Verification items for the finished model (mm, model axes). A direction names the side the tool comes from. Coordinates: 2 decimals unless noted, no trailing zeros. Answer as CSV lines item,"result". Start each with the question number.
1. Mould release check, pull along Y, two halves, no side actions. Record for faces 1 (the flat face through (45, -42.679, -10)), 2 (the flat face through (20, -66, -50.8)), 3 (the cylindrical face through (11.75, -57.24, 6.37)): pulls with the +Y half, pulls with the -Y half, needs draft (parallel to the pull), parting line crosses it, or undercut.
2. Set-up check for faces 4 (the cylindrical face through (11.569, -65.792, 6.368)), 5 (the flat face through (16.233, -34, -45)), 6 (the flat face through (3, -61.729, -58)), 7 (the cylindrical face through (19.898, -68.856, 10.196)): record each of +Z, -Z, +X, -X, +Y, -Y from which the full face is reachable in a straight line by a thin tool's end or side.
3. Section check A-A (y = -59.5). Count the separate pieces of the cut face and the enclosed holes in it, and give its area (3 significant figures).
4. Go/stop test with flat-tipped pins: pin 1 (8.5 mm diameter, centred on x = 46, z = -13, fed in from -Y); pin 2 (3.5 mm diameter, centred on x = 28.93, y = -29.98, fed in from -Z); pin 3 (3.5 mm diameter, centred on x = 18.5, y = -66.5, fed in from +Z); pin 4 (6 mm diameter, centred on x = 24.5, z = -47, fed in from -Y). Record where each tip stops, or that it passes through.
5. Material ranges on L1, parallel to Y at x = 25, z = -46.5; L2, parallel to X at y = -54, z = -55; L3, parallel to Z at x = 7.5, y = -51.5, recorded low to high. Write a range as [from, to].
from build123d import *

# Parameters (mm, degrees)
SKETCH1_W            = 50.8
SKETCH1_H            = 76.2
BOSS_EXTRUDE1_DEPTH  = 12.7
SKETCH3_R            = 2.032
CUT_EXTRUDE1_DEPTH   = 12.7
SKETCH17_W           = 7.62
SKETCH17_H           = 76.2
BOSS_EXTRUDE13_DEPTH = 68.58
SKETCH18_W           = 3.81
SKETCH18_H           = 19.05
BOSS_EXTRUDE14_DEPTH = 43.18
SKETCH19_W           = 29.21
SKETCH19_H           = 19.05
BOSS_EXTRUDE15_DEPTH = 43.18
SKETCH4_R            = 4.064
CUT_EXTRUDE5_DEPTH   = 125.729995039
CUT_EXTRUDE6_START   = -5.08
SKETCH21_R           = 11.176
SKETCH21_R_2         = 4.064
CUT_EXTRUDE6_DEPTH   = 5.08
SKETCH22_R           = 11.176
SKETCH22_R_2         = 4.064
CUT_EXTRUDE7_DEPTH   = 5.08
SKETCH23_W           = 19.05
SKETCH23_H           = 38.1
CUT_EXTRUDE8_DEPTH   = 115.424594585
SKETCH26_W           = 17.78
SKETCH26_H           = 46.99
BOSS_EXTRUDE16_DEPTH = 57.15
SKETCH28_W           = 50.8
SKETCH28_H           = 81.28
BOSS_EXTRUDE18_DEPTH = 3.81
SKETCH35_R           = 4.064
CUT_EXTRUDE10_DEPTH  = 125.729995039
SKETCH32_R           = 2.032
CUT_EXTRUDE12_DEPTH  = 9.525
SKETCH41_R           = 2.032
CUT_EXTRUDE14_DEPTH  = 9.525
SKETCH43_R           = 3.96875
CUT_EXTRUDE15_DEPTH  = 4.7625
SKETCH46_R           = 3.937
CUT_EXTRUDE17_DEPTH  = 3.048
SKETCH48_R           = 2.54
CUT_EXTRUDE18_DEPTH  = 25.908
SKETCH49_W           = 50.8
SKETCH49_H           = 4.744734857
CUT_EXTRUDE19_DEPTH  = 92.202
CUT_EXTRUDE20_DEPTH  = 92.202
SKETCH52_W           = 50.8
SKETCH52_H           = 6.844747076
CUT_EXTRUDE21_DEPTH  = 62.484
CUT_EXTRUDE22_DEPTH  = 23.876
FILLET1_R            = 6.35
FILLET2_R            = 6.35
FILLET3_R            = 6.35
FILLET4_R            = 6.35
FILLET5_R            = 6.35
FILLET6_R            = 6.35
FILLET7_R            = 6.35
FILLET8_R            = 6.35


with BuildPart() as part:
    # Sketch1 → Boss-Extrude1 (new body)
    with BuildSketch(Plane.XY):
        with Locations((23.853164533, -42.679075546)):
            Rectangle(SKETCH1_W, SKETCH1_H)
    extrude(amount=BOSS_EXTRUDE1_DEPTH)

    # Sketch3 → Cut-Extrude1 (cut)
    with BuildSketch(Plane.XY.offset(12.7)):
        with Locations((28.933164533, -42.679075546)):
            Circle(SKETCH3_R)
        with Locations((28.933164533, -29.979075546)):
            Circle(SKETCH3_R)
        with Locations((28.933164533, -17.279075546)):
            Circle(SKETCH3_R)
    extrude(amount=-CUT_EXTRUDE1_DEPTH, mode=Mode.SUBTRACT)

    # Sketch17 → Boss-Extrude13 (add)
    with BuildSketch(Plane(origin=(0, 0, 0), x_dir=(-1, 0, 0), z_dir=(0, 0, -1))):
        with Locations((-45.443164533, -42.679075546)):
            Rectangle(SKETCH17_W, SKETCH17_H)
    extrude(amount=BOSS_EXTRUDE13_DEPTH)

    # Sketch18 → Boss-Extrude14 (add)
    with BuildSketch(Plane.ZY.offset(-41.633164533)):
        with Locations((-66.675, -71.254075546)):
            Rectangle(SKETCH18_W, SKETCH18_H)
    extrude(amount=BOSS_EXTRUDE14_DEPTH)

    # Sketch19 → Boss-Extrude15 (add)
    with BuildSketch(Plane.ZY.offset(-41.633164533)):
        with Locations((-36.195, -71.254075546)):
            Rectangle(SKETCH19_W, SKETCH19_H)
    extrude(amount=BOSS_EXTRUDE15_DEPTH)

    # Sketch4 → Cut-Extrude5 (cut, through all)
    with BuildSketch(Plane.XY.offset(12.7)):
        with Locations((11.661164533, -61.30266317)):
            Circle(SKETCH4_R)
    extrude(amount=-CUT_EXTRUDE5_DEPTH, mode=Mode.SUBTRACT)

    # Sketch21 → Cut-Extrude6 (cut)
    with BuildSketch(Plane(origin=(0, 0, 0), x_dir=(-1, 0, 0), z_dir=(0, 0, -1)).offset(CUT_EXTRUDE6_START)):
        with Locations((-11.661164533, -61.30266317)):
            Circle(SKETCH21_R)
        with Locations(Location((-11.661164533, -61.30266317, 0), (0, 0, 180))):
            Circle(SKETCH21_R_2, mode=Mode.SUBTRACT)
    extrude(amount=CUT_EXTRUDE6_DEPTH, mode=Mode.SUBTRACT)

    # Sketch22 → Cut-Extrude7 (cut)
    with BuildSketch(Plane.XY.offset(12.7)):
        with Locations(Location((11.661164533, -61.30266317, 0), (0, 0, 180))):
            Circle(SKETCH22_R)
        with Locations((11.661164533, -61.30266317)):
            Circle(SKETCH22_R_2, mode=Mode.SUBTRACT)
    extrude(amount=-CUT_EXTRUDE7_DEPTH, mode=Mode.SUBTRACT)

    # Sketch23 → Cut-Extrude8 (cut, through all)
    with BuildSketch(Plane.ZY.offset(-41.633164533)):
        with Locations((-9.525, -61.729075546)):
            Rectangle(SKETCH23_W, SKETCH23_H)
    extrude(amount=-CUT_EXTRUDE8_DEPTH, mode=Mode.SUBTRACT)

    # Sketch26 → Boss-Extrude16 (add)
    with BuildSketch(Plane(origin=(0, -61.729075546, 0), x_dir=(1, 0, 0), z_dir=(0, 1, 0))):
        with Locations((7.343164533, 45.085)):
            Rectangle(SKETCH26_W, SKETCH26_H)
    extrude(amount=BOSS_EXTRUDE16_DEPTH)

    # Sketch28 → Boss-Extrude18 (add)
    with BuildSketch(Plane(origin=(0, -4.579075546, 0), x_dir=(1, 0, 0), z_dir=(0, 1, 0))):
        with Locations((23.853164533, 27.94)):
            Rectangle(SKETCH28_W, SKETCH28_H)
    extrude(amount=BOSS_EXTRUDE18_DEPTH)

    # Sketch35 → Cut-Extrude10 (cut, through all)
    with BuildSketch(Plane.XY.offset(12.7)):
        with Locations((11.661164533, -61.729075546)):
            Circle(SKETCH35_R)
    extrude(amount=-CUT_EXTRUDE10_DEPTH, mode=Mode.SUBTRACT)

    # Sketch32 → Cut-Extrude12 (cut)
    with BuildSketch(Plane(origin=(49.253164533, 0, 0), x_dir=(0, 0, -1), z_dir=(1, 0, 0))):
        with Locations(Location((-3.81, -36.329075546, 0), (0, 0, 90))):
            Circle(SKETCH32_R)
        with Locations(Location((-3.81, -10.929075546, 0), (0, 0, 90))):
            Circle(SKETCH32_R)
    extrude(amount=-CUT_EXTRUDE12_DEPTH, mode=Mode.SUBTRACT)

    # Sketch41 → Cut-Extrude14 (cut)
    with BuildSketch(Plane.ZY.offset(-41.633164533)):
        with Locations(Location((-57.658, -10.929075546, 0), (0, 0, 270))):
            Circle(SKETCH41_R)
        with Locations(Location((-57.658, -60.459075546, 0), (0, 0, 270))):
            Circle(SKETCH41_R)
    extrude(amount=-CUT_EXTRUDE14_DEPTH, mode=Mode.SUBTRACT)

    # Sketch43 → Cut-Extrude15 (cut)
    with BuildSketch(Plane.ZY.offset(-41.633164533)):
        with Locations(Location((-57.658, -10.929075546, 0), (0, 0, 270))):
            Circle(SKETCH43_R)
        with Locations(Location((-57.658, -60.459075546, 0), (0, 0, 270))):
            Circle(SKETCH43_R)
    extrude(amount=-CUT_EXTRUDE15_DEPTH, mode=Mode.SUBTRACT)

    # Sketch46 → Cut-Extrude17 (cut)
    with BuildSketch(Plane(origin=(0, 0, 0), x_dir=(-1, 0, 0), z_dir=(0, 0, -1))):
        with Locations((-28.933164533, -42.679075546)):
            Circle(SKETCH46_R)
    extrude(amount=-CUT_EXTRUDE17_DEPTH, mode=Mode.SUBTRACT)

    # Sketch48 → Cut-Extrude18 (cut)
    with BuildSketch(Plane.ZY.offset(1.546835467)):
        with Locations(Location((-57.658, -10.929075546, 0), (0, 0, 270))):
            Circle(SKETCH48_R)
    extrude(amount=-CUT_EXTRUDE18_DEPTH, mode=Mode.SUBTRACT)

    # Sketch49 → Cut-Extrude19 (cut)
    with BuildSketch(Plane.XY.offset(12.7)):
        with Locations((23.853164533, -78.406708118)):
            Rectangle(SKETCH49_W, SKETCH49_H)
    extrude(amount=-CUT_EXTRUDE19_DEPTH, mode=Mode.SUBTRACT)

    # Sketch51 → Cut-Extrude20 (cut)
    with BuildSketch(Plane.XY.offset(12.7)):
        Polygon((13.530749107, -0.769075546), (-1.546835467, -54.869608678), (-1.546835467, -0.769075546), align=None)
    extrude(amount=-CUT_EXTRUDE20_DEPTH, mode=Mode.SUBTRACT)

    # Sketch52 → Cut-Extrude21 (cut)
    with BuildSketch(Plane(origin=(0, 0, -68.58), x_dir=(-1, 0, 0), z_dir=(0, 0, -1))):
        with Locations((-23.853164533, -72.611967151)):
            Rectangle(SKETCH52_W, SKETCH52_H)
    extrude(amount=-CUT_EXTRUDE21_DEPTH, mode=Mode.SUBTRACT)

    # Sketch53 → Cut-Extrude22 (cut)
    with BuildSketch(Plane.XY.offset(12.7)):
        Polygon((23.853164533, -76.034340689), (49.253164533, -47.175169833), (49.253164533, -76.034340689), align=None)
    extrude(amount=-CUT_EXTRUDE22_DEPTH, mode=Mode.SUBTRACT)

    # Fillet1
    fillet1_edges = [part.edges().sort_by_distance(p)[0] for p in [
        (-1.546835467, -54.869608678, -45.085),
    ]]
    fillet(fillet1_edges, radius=FILLET1_R)

    # Fillet2
    # the kernel refuses this fillet: 6.35 mm, written as the material it takes off along each edge
    with BuildSketch(Plane(origin=(13.530749107, -0.769075546, 24.755694059), x_dir=(-0.26846462888250333, -0.9632895426812126, 0), z_dir=(0, 0, -1))) as fillet2_piece_1:
        with BuildLine():
            CenterArc((FILLET2_R * 0.759413798972, -FILLET2_R), FILLET2_R, 90, 74.427076266)
            Line((-FILLET2_R * 0.203875743709, -FILLET2_R * 0.731535371117), (0, 0))
            Line((0, 0), (FILLET2_R * 0.759413798972, 0))
        make_face()
    extrude(amount=105.391388117, mode=Mode.SUBTRACT)

    # Fillet3
    fillet3_edges = [part.edges().sort_by_distance(p)[0] for p in [
        (-1.546835467, -54.869608678, 6.35),
    ]]
    fillet(fillet3_edges, radius=FILLET3_R)

    # Fillet4
    fillet4_edges = [part.edges().sort_by_distance(p)[0] for p in [
        (49.253164533, -0.769075546, -27.94),
    ]]
    fillet(fillet4_edges, radius=FILLET4_R)

    # Fillet5
    fillet5_edges = [part.edges().sort_by_distance(p)[0] for p in [
        (49.253164533, -47.175169833, 6.35),
    ]]
    fillet(fillet5_edges, radius=FILLET5_R)

    # Fillet6
    fillet6_edges = [part.edges().sort_by_distance(p)[0] for p in [
        (-1.546835467, -76.034340689, 6.35),
        (23.853164533, -76.034340689, 6.35),
    ]]
    fillet(fillet6_edges, radius=FILLET6_R)

    # Fillet7
    fillet7_edges = [part.edges().sort_by_distance(p)[0] for p in [
        (-1.546835467, -69.189593613, -66.675),
        (-1.546835467, -69.189593613, -36.195),
    ]]
    fillet(fillet7_edges, radius=FILLET7_R)

    # Fillet8
    fillet8_edges = [part.edges().sort_by_distance(p)[0] for p in [
        (49.253164533, -69.189593613, -43.815),
    ]]
    fillet(fillet8_edges, radius=FILLET8_R)


solid = part.part
Evaluation:
1,face 1,"pulls with the -Y half"
1,face 2,"needs draft"
1,face 3,"undercut"
2,face 4,"+Z, -Z"
2,face 5,"-Z"
2,face 6,"-X, -Y"
2,face 7,"+Z"
3,separate pieces,"6"
3,enclosed holes,"0"
3,area,"1,110 mm²"
4,pin 1,"stops at y = -42.68"
4,pin 2,"passes through"
4,pin 3,"stops at z = 7.62"
4,pin 4,"stops at y = -69.19"
5,L1,"y = [-69.19, -61.73], [-4.58, -0.77]"
5,L2,"x = [-1.3, 16.23], [41.63, 49.25]"
5,L3,"z = [-68.58, -21.59], [5.08, 7.62]"
